Work out the finished part from the listing and answer in its coordinate system (mm). A direction names the side the tool comes from. Coordinates: 2 decimals unless noted, no trailing zeros. Loops run counter-clockwise (first coordinate to the right, second up) from the corner with the lowest first, then second, coordinate; pieces in that order, holes last. Notation, with made-up numbers: (88, 48.25) -> (137, 48.25) arc R30 cw to (137, 77.25) -> close; hole circle Ø10 at (5.5, 39.5). An arc over 180 degrees is marked (long way). Use a Markdown table: item, result.
from build123d import *

# Parameters (mm, degrees)
BOSS_EXTRUDE1_DEPTH         = 6.35
F_3_4_0_75_DIAMETER_HOLE1_D = 19.05
F_10_0_10_DIAMETER_HOLE1_D  = 10
F_5_8_DIAMETER_HOLE2_D      = 15.875
CUT_EXTRUDE1_REACH          = 205.594
FILLET1_R                   = 35
FILLET3_R                   = 35
FILLET4_R                   = 20
FILLET6_R                   = 40
SKETCH22_R                  = 2.65
CUT_EXTRUDE2_DEPTH          = 10
SKETCH24_R                  = 2.65
CUT_EXTRUDE3_DEPTH          = 10


with BuildPart() as part:
    # Sketch1 → Boss-Extrude1 (new body)
    with BuildSketch(Plane(origin=(0, 0, 0), x_dir=(0, 0, -1), z_dir=(1, 0, 0))):
        with BuildLine():
            Line((-60.717143143, 0), (60.717143143, 0))
            ThreePointArc((60.717143143, 0), (94.584407895, 9.944020783), (67.452353804, 32.521151068))
            Line((67.452353804, 32.521151068), (-134.404938559, 119.878311848))
            ThreePointArc((-134.404938559, 119.878311848), (-155.966181949, 122.347168224), (-149.752887031, 101.553480851))
            Line((-149.752887031, 101.553480851), (-94.55805454, 18.181208272))
            ThreePointArc((-94.55805454, 18.181208272), (-84.465516954, -3.618285637), (-60.717143143, 0))
        make_face()
    extrude(amount=BOSS_EXTRUDE1_DEPTH)

    # 3/4 (0.75) Diameter Hole1 (through all)
    with Locations(Plane(origin=(6.35, 0, 0), x_dir=(0, 0, -1), z_dir=(1, 0, 0))):
        with Locations((75, 14)):
            Hole(F_3_4_0_75_DIAMETER_HOLE1_D / 2)

    # Ø10.0 (10) Diameter Hole1 (through all)
    with Locations(Plane(origin=(6.35, 0, 0), x_dir=(0, 0, -1), z_dir=(1, 0, 0))):
        with Locations((-146, 114)):
            Hole(F_10_0_10_DIAMETER_HOLE1_D / 2)

    # Ø5/8" Diameter Hole2 (through all)
    with Locations(Plane(origin=(6.35, 0, 0), x_dir=(0, 0, -1), z_dir=(1, 0, 0))):
        with Locations((-75, 14)):
            Hole(F_5_8_DIAMETER_HOLE2_D / 2)

    # Sketch8 → Cut-Extrude1 (cut, up to next)
    with BuildSketch(Plane(origin=(6.35, 0, 0), x_dir=(0, 0, -1), z_dir=(1, 0, 0)), mode=Mode.PRIVATE) as cut_extrude1_sk1:
        with BuildLine():
            Line((-52.98768213, 32.027989609), (-48.791838571, 52.287736349))
            ThreePointArc((-48.791838571, 52.287736349), (-43.609219792, 59.133963583), (-35.027937054, 59.43719837))
            Line((-35.027937054, 59.43719837), (22.864909862, 34.383088722))
            ThreePointArc((22.864909862, 34.383088722), (27.230289645, 25.979007794), (19.886136685, 20))
            Line((19.886136685, 20), (-43.195478183, 20))
            ThreePointArc((-43.195478183, 20), (-50.950473221, 23.686518238), (-52.98768213, 32.027989609))
        make_face()
    cut_extrude1_tool1 = extrude(cut_extrude1_sk1.sketch, amount=-CUT_EXTRUDE1_REACH, mode=Mode.PRIVATE) & part.part
    # Sketch8 → Cut-Extrude1 (cut, up to next)
    with BuildSketch(Plane(origin=(6.35, 0, 0), x_dir=(0, 0, -1), z_dir=(1, 0, 0)), mode=Mode.PRIVATE) as cut_extrude1_sk2:
        with BuildLine():
            Line((-75.95726339, 42.34340423), (-63.166421785, 57.61515284))
            ThreePointArc((-63.166421785, 57.61515284), (-61.101947711, 66.340863059), (-66.861018022, 73.213503103))
            Line((-66.861018022, 73.213503103), (-119.037006728, 95.793545572))
            ThreePointArc((-119.037006728, 95.793545572), (-123.11030371, 94.828752024), (-123.345509052, 90.649367698))
            Line((-123.345509052, 90.649367698), (-91.961866267, 43.244103424))
            ThreePointArc((-91.961866267, 43.244103424), (-84.185443207, 38.780101137), (-75.95726339, 42.34340423))
        make_face()
    cut_extrude1_tool2 = extrude(cut_extrude1_sk2.sketch, amount=-CUT_EXTRUDE1_REACH, mode=Mode.PRIVATE) & part.part
    add(cut_extrude1_tool1.solids().sort_by_distance((6.35, 35.497015, 18.727672))[0], mode=Mode.SUBTRACT)
    add(cut_extrude1_tool2.solids().sort_by_distance((6.35, 67.079595, 89.97893))[0], mode=Mode.SUBTRACT)

    # Fillet1
    fillet1_edges = [part.edges().sort_by_distance(p)[0] for p in [
        (3.175, 18.181208272, 94.55805454),
    ]]
    fillet(fillet1_edges, radius=FILLET1_R)

    # Fillet3
    fillet3_edges = [part.edges().sort_by_distance(p)[0] for p in [
        (3.175, 32.521151068, -67.452353804),
        (3.175, 0, -60.717143143),
    ]]
    fillet(fillet3_edges, radius=FILLET3_R)

    # Fillet4
    fillet4_edges = [part.edges().sort_by_distance(p)[0] for p in [
        (3.175, 101.553480851, 149.752887031),
        (3.175, 119.878311848, 134.404938559),
    ]]
    fillet(fillet4_edges, radius=FILLET4_R)

    # Fillet6
    fillet6_edges = [part.edges().sort_by_distance(p)[0] for p in [
        (3.175, 0, 60.717143143),
    ]]
    fillet(fillet6_edges, radius=FILLET6_R)

    # Sketch22 → Cut-Extrude2 (cut)
    with BuildSketch(Plane(origin=(6.35, 0, 0), x_dir=(0, 0, -1), z_dir=(1, 0, 0))):
        with Locations((60.644779113, 26.750227475)):
            Circle(SKETCH22_R)
    extrude(amount=-CUT_EXTRUDE2_DEPTH, mode=Mode.SUBTRACT)

    # Sketch24 → Cut-Extrude3 (cut)
    with BuildSketch(Plane(origin=(6.35, 0, 0), x_dir=(0, 0, -1), z_dir=(1, 0, 0))):
        with Locations((42.966527297, 34.400790246)):
            Circle(SKETCH24_R)
    extrude(amount=-CUT_EXTRUDE3_DEPTH, mode=Mode.SUBTRACT)


solid = part.part
Q1. Section A-A on z = 109 is taken. Determine the outline of the cut face in (x, y).
Solved:
| item | result |
|---|---|
| outline | (0, 40) -> (6.35, 40) -> (6.35, 68.98) -> (0, 68.98) -> close; (0, 91.45) -> (6.35, 91.45) -> (6.35, 108.88) -> (0, 108.88) -> close |
Q2. For faces 5 (the flat face through (0, 46, 51)), 6 (the flat face through (3.219, 47.086, 6.487)), 7 (the cylindrical face through (3.22, -1.04, 57.91)), determine the directions among +Z, -Z, +X, -X, +Y, -Y from which every point of the face is accessible in a straight line to the end or side of a thin tool.
Solved:
| item | result |
|---|---|
| face 5 | +Z, -Z, -X, +Y, -Y |
| face 6 | +X, -X |
| face 7 | +X, -X, -Y |
Q3. Section C-C on x = 1.75 is taken. State how many separate pieces and enclosed holes the cut face has, and give its area (3 significant figures).
Solved:
| item | result |
|---|---|
| separate pieces | 1 |
| enclosed holes | 7 |
| area | 10,700 mm² |
Q4. Given pin 1 Ø1.5 at (x, y) = (1, 23) entering from -Z; pin 2 Ø1.9 at (x, z) = (2, -21) entering from -Y; pin 3 Ø2 at (x, y) = (5, 47) entering from -Z; pin 4 Ø8 at (y, z) = (114, 146) entering from -X, each flat-ended and moving along its own axis, determine where each tip first touches the part or whether it passes through.
Solved:
| item | result |
|---|---|
| pin 1 | z = -93.22 |
| pin 2 | y = 0 |
| pin 3 | z = -36.31 |
| pin 4 | through |
Q5. Section B-B on y = 114 is taken. Determine the outline of the cut face in (x, z).
Solved:
| item | result |
|---|---|
| outline | (0, 120.82) -> (6.35, 120.82) -> (6.35, 141) -> (0, 141) -> close; (0, 151) -> (6.35, 151) -> (6.35, 159) -> (0, 159) -> close |
Q6. Determine the mould class of faces 1 (the cylindrical face through (3.22, -0.94, -58.08)), 2 (the flat face through (3.131, 76.677, 34.579)), 3 (the cylindrical face through (3.219, 35.197, -45.494)), 4 (the cylindrical face through (3.131, 9.441, -94.474)) for opening direction Y: pulls with the +Y half, pulls with the -Y half, needs draft (parallel to the pull), parting line crosses it, or undercut.
Solved:
| item | result |
|---|---|
| face 1 | pulls with the -Y half |
| face 2 | pulls with the +Y half |
| face 3 | undercut |
| face 4 | parting line crosses it |
Q7. Consider line 1 (Z direction, x = 2, y = 21) (3 decimals); line 2 (Y direction, x = 5, z = -75) (3 decimals); line 3 (Y direction, x = 1.5, z = 105). Determine where each line is inside the solid, lowest interval first. Write a range as [from, to].
Solved:
| item | result |
|---|---|
| line 1 | [-93.735, -81.46], [-68.54, -23.628], [47.554, 71.258], [78.742, 97.24] |
| line 2 | [-6, 4.475], [23.525, 34] |
| line 3 | [33.95, 62.94], [89.72, 107.15] |
